from build123d import *

# Parameters (mm, degrees)
F0_W     = 127
F0_H     = 76.2
F0_W_2   = 114.3
F0_H_2   = 63.5
F1_DEPTH = 31.75
F3_DEPTH = 101.6
F4_R     = 7.336255
F5_DEPTH = 127


with BuildPart() as f1:
    # F0 (on Top) → F1 (new body, symmetric)
    with BuildSketch(Plane.XY):
        Rectangle(F0_W, F0_H)
        Rectangle(F0_W_2, F0_H_2, mode=Mode.SUBTRACT)
    extrude(amount=F1_DEPTH, both=True)

    # F2 (on face) → F3 (cut)
    with BuildSketch(Plane.XZ.offset(38.1)):
        Polygon((30.48, 31.75), (-30.48, 31.75), (-30.48, 0), (0, 0), (30.48, 0), align=None)
    extrude(amount=-F3_DEPTH, mode=Mode.SUBTRACT)

    # F4 (on face) → F5 (cut)
    with BuildSketch(Plane.YZ.offset(63.5)):
        Circle(F4_R)
    extrude(amount=-F5_DEPTH, mode=Mode.SUBTRACT)


solid = f1.part
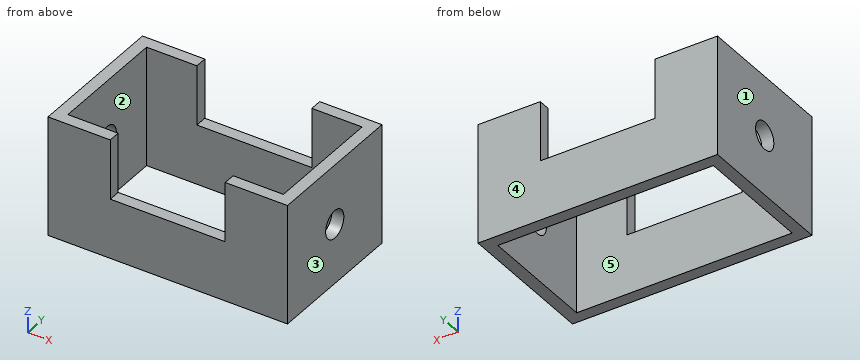
Could you check a few things on this model? Use its own coordinates, in mm. Face numbers are marked on the shaded views. A direction names the side the tool comes from. Give positions to 0.01 mm unless a question says otherwise; leave off trailing zeros. Order: outer loops, then holes, each group sorted by start corner. A loop starts at its lowest first (then second) coordinate and runs counter-clockwise, first axis right, second up.
1. Will this pin go through, and if not, where does the flat tip stop? P1, Ø5, axis at x = -4.5, y = 36, coming from the +Z side.
2. We'd pull the mould along Y, two halves only. Please class the marked faces 3, 4 and 5: pulls with the +Y half, pulls with the -Y half, needs draft (parallel to the pull), parting line crosses it, or undercut.
3. I need wall thicknesses on L1, parallel to Z at x = 61.75, y = 0; L2, parallel to Y at x = 57, z = -9; L3, parallel to X at y = 13, z = 17. Which ranges of each line are inside material? Lowest first, please.
4. For the marked faces 1 and 2, which set-ups out of +Z, -Z, +X, -X, +Y, -Y let a thin tool reach every point of the face, with its end or its side?
5. Suppose I cut it at B-B (x = 51.5). List the corners of the cut face in (y, z) for me.
6. Suppose I cut it at A-A (y = 0). List the corners of the cut face in (x, z) for me, plus the area to 3 significant figures.
7. Suppose I cut it at C-C (z = -9.5). List the corners of the cut face in (x, y) for me.
8. Suppose I cut it at D-D (y = -21.5). List the corners of the cut face in (x, z) for me.
Solved:
1. P1: stops at z = 0
2. face 3: needs draft
2. face 4: pulls with the +Y half
2. face 5: undercut
3. L1: z = -31.75 to -7.34, 7.34 to 31.75
3. L2: y = -38.1 to -31.75, 31.75 to 38.1
3. L3: x = -63.5 to -57.15, 57.15 to 63.5
4. face 1: +Z, -Z, -X, +Y, -Y
4. face 2: +Z, -Z
5. outline: (-38.1, -31.75) - (-31.75, -31.75) - (-31.75, 31.75) - (-38.1, 31.75) - close; (31.75, -31.75) - (38.1, -31.75) - (38.1, 31.75) - (31.75, 31.75) - close
6. outline: (-63.5, -31.75) - (-57.15, -31.75) - (-57.15, -7.34) - (-63.5, -7.34) - close; (-63.5, 7.34) - (-57.15, 7.34) - (-57.15, 31.75) - (-63.5, 31.75) - close; (57.15, -31.75) - (63.5, -31.75) - (63.5, -7.34) - (57.15, -7.34) - close; (57.15, 7.34) - (63.5, 7.34) - (63.5, 31.75) - (57.15, 31.75) - close
6. area: 620 mm2
7. outline: (-63.5, -38.1) - (63.5, -38.1) - (63.5, 38.1) - (-63.5, 38.1) - close; hole (-57.15, -31.75) - (57.15, -31.75) - (57.15, 31.75) - (-57.15, 31.75) - close
8. outline: (-63.5, -31.75) - (-57.15, -31.75) - (-57.15, 31.75) - (-63.5, 31.75) - close; (57.15, -31.75) - (63.5, -31.75) - (63.5, 31.75) - (57.15, 31.75) - close
